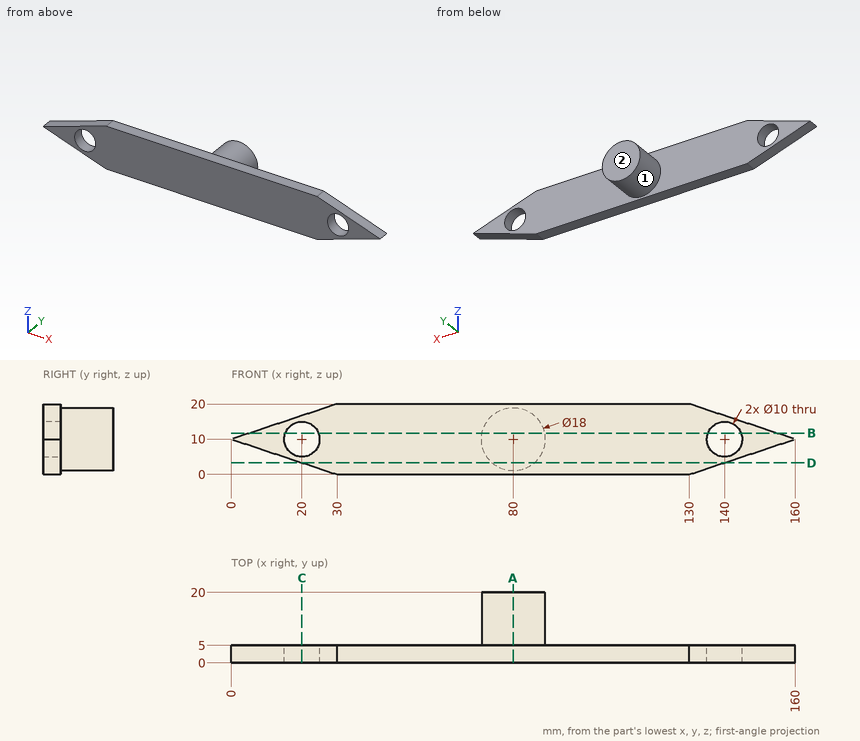
Source: three-view drawing plus pictorial views. Frame: mm from the lowest corner of the part. A direction names the side the tool comes from. Round coordinates to 2 decimals unless told otherwise and drop trailing zeros. Order: outer loops, then holes, each group sorted by start corner. A loop starts at its lowest first (then second) coordinate and runs counter-clockwise, first axis right, second up. Notation, with made-up numbers: (3.25, -32.75) - (19.25, -32.75) arc R19 ccw to (19.25, 3.25) - close; hole circle Ø7 at (13, 4.5). An arc over 180 degrees is marked (long way). Answer in a Markdown table with one row per item.
Item 1: Section query A-A (x = 80). Return the cut outline in (y, z), then the cut area to 3 significant figures.
Model answer:
| item | result |
|---|---|
| outline | (0, 0) - (5, 0) - (5, 1) - (20, 1) - (20, 19) - (5, 19) - (5, 20) - (0, 20) - close |
| area | 370 mm² |
Item 2: Pin query (flat end, axial travel): pin 1 (6 mm diameter, centred on x = 89, z = 8, fed in from +Y); pin 2 (6 mm diameter, centred on y = 15.5, z = 9, fed in from -X); pin 3 (1.5 mm diameter, centred on y = 11.5, z = 13, fed in from -X); pin 4 (3 mm diameter, centred on y = 11.5, z = 3.5, fed in from +X). Return the tip coordinate at first contact, or that it passes through.
Model answer:
| item | result |
|---|---|
| pin 1 | stops at y = 20 |
| pin 2 | stops at x = 71 |
| pin 3 | stops at x = 71.29 |
| pin 4 | stops at x = 87.48 |
Item 3: Reachability of the marked faces 1 and 2 from +Z, -Z, +X, -X, +Y, -Y: full face, straight path, thin tool, end or side. Return the list, or none.
Model answer:
| item | result |
|---|---|
| face 1 | +Y |
| face 2 | +Z, -Z, +X, -X, +Y |
Item 4: Section query D-D (z = 3.25). Return the cut outline in (x, y).
Model answer:
| item | result |
|---|---|
| outline | (20.25, 0) - (139.75, 0) - (139.75, 5) - (85.95, 5) - (85.95, 20) - (74.05, 20) - (74.05, 5) - (20.25, 5) - close |
Item 5: Section query C-C (x = 20). Return the cut outline in (y, z).
Model answer:
| item | result |
|---|---|
| outline | (0, 3.33) - (5, 3.33) - (5, 5) - (0, 5) - close; (0, 15) - (5, 15) - (5, 16.67) - (0, 16.67) - close |
Item 6: Section query B-B (z = 11.75). Return the cut outline in (x, y).
Model answer:
| item | result |
|---|---|
| outline | (5.25, 0) - (15.32, 0) - (15.32, 5) - (5.25, 5) - close; (24.68, 0) - (135.32, 0) - (135.32, 5) - (88.83, 5) - (88.83, 20) - (71.17, 20) - (71.17, 5) - (24.68, 5) - close; (144.68, 0) - (154.75, 0) - (154.75, 5) - (144.68, 5) - close |
Item 7: Line query: line 1 (Y direction, x = 48, z = 11); line 2 (Z direction, x = 80.5, y = 17.75); line 3 (Z direction, x = 140, y = 2.75). Output: solid intervals per line, ascending.
Model answer:
| item | result |
|---|---|
| line 1 | y = 0 to 5 |
| line 2 | z = 1.01 to 18.99 |
| line 3 | z = 3.33 to 5, 15 to 16.67 |
